Source: CAD feature listing. Evaluate the final solid. Frame: model axes, mm. Give positions to 0.01 mm unless a question says otherwise; leave off trailing zeros. Loops run counter-clockwise (first coordinate to the right, second up) from the corner with the lowest first, then second, coordinate; pieces in that order, holes last. Notation, with made-up numbers: M -16,-20.5 L 11,-20.5 A32 ccw 11,18.5 Z; hole C -10,4.5 d7. An arc over 180 degrees is marked long. Answer in a Markdown table with one row per item.
```python
from build123d import *

# Parameters (mm, degrees)
BOSS_EXTRUDE1_DEPTH = 10
SKETCH2_R           = 5
CUT_EXTRUDE1_DEPTH  = 10


with BuildPart() as part:
    # Sketch1 → Boss-Extrude1 (new body)
    with BuildSketch(Plane.XY):
        with BuildLine():
            Line((-201.501450472, -50.838763567), (172.498549528, -50.838763567))
            Line((172.498549528, -50.838763567), (188.762005495, -34.5753076))
            Line((188.762005495, -34.5753076), (148.240026218, 28.535461651))
            ThreePointArc((148.240026218, 28.535461651), (147.2053445, 29.880442481), (146.412969402, 31.381002841))
            Line((146.412969402, 31.381002841), (137.047280897, 53.478149236))
            Line((137.047280897, 53.478149236), (5.239743471, 86.985955455))
            Line((5.239743471, 86.985955455), (-43.250387022, 55.851553414))
            ThreePointArc((-43.250387022, 55.851553414), (-53.613723576, 40.938672068), (-71.486708656, 37.721658093))
            Line((-71.486708656, 37.721658093), (-139.427338947, 0))
            Line((-139.427338947, 0), (-201.501450472, -50.838763567))
        make_face()
    extrude(amount=BOSS_EXTRUDE1_DEPTH)

    # Sketch2 → Cut-Extrude1 (cut)
    with BuildSketch(Plane.XY.offset(10)):
        with Locations((5.274158071, 0)):
            Circle(SKETCH2_R)
    extrude(amount=-CUT_EXTRUDE1_DEPTH, mode=Mode.SUBTRACT)


solid = part.part
```
1) Section C-C, the plane y = -22. Return loops of the section in (x, z), then the cut area to 3 significant figures.
Reply:
| item | result |
|---|---|
| outline | M -166.29,0 L 180.69,0 L 180.69,10 L -166.29,10 Z |
| area | 3,470 mm² |
2) Pull-direction query (X, two-part tool) for faces 1 (the cylindrical face through (-53.395, 41.081, 4.93)), 2 (the cylindrical face through (1.306, -3.042, 5.07)), 3 (the flat face through (-18.666, 71.637, 4.93)), 4 (the flat face through (34, 4, 10)); classes: released by +X, released by -X, zero draft, split by the parting line, or undercut.
Reply:
| item | result |
|---|---|
| face 1 | undercut |
| face 2 | undercut |
| face 3 | released by -X |
| face 4 | zero draft |
3) Section B-B, the plane x = 57. Return loops of the section in (y, z).
Reply:
| item | result |
|---|---|
| outline | M -50.84,0 L 73.83,0 L 73.83,10 L -50.84,10 Z |
4) Pin query (flat end, axial travel): pin 1 Ø4 at (x, y) = (133.5, 56) entering from +Z; pin 2 Ø2 at (y, z) = (-3.5, 3.5) entering from +X; pin 3 Ø6 at (y, z) = (-13.5, 8.5) entering from +X. Return the tip coordinate at first contact, or that it passes through.
Reply:
| item | result |
|---|---|
| pin 1 | stops at z = 10 |
| pin 2 | stops at x = 169.45 |
| pin 3 | stops at x = 177.16 |
5) Section A-A, the plane z = 3.75. Return loops of the section in (x, y).
Reply:
| item | result |
|---|---|
| outline | M -201.5,-50.84 L 172.5,-50.84 L 188.76,-34.58 L 148.24,28.54 A10 cw 146.41,31.38 L 137.05,53.48 L 5.24,86.99 L -43.25,55.85 A23.73 cw -71.49,37.72 L -139.43,0 Z; hole C 5.27,0 d10 |
6) Material intervals for L1, parallel to Y at x = 4, z = 6; L2, parallel to X at y = -31, z = 6.25; L3, parallel to Y at x = 157.5, z = 0.5, sorted ascending.
Reply:
| item | result |
|---|---|
| L1 | y = -50.84 to -4.83, 4.83 to 86.19 |
| L2 | x = -177.28 to 186.47 |
| L3 | y = -50.84 to 14.11 |
